Verification items for the finished model (mm, model axes). A direction names the side the tool comes from. Coordinates: 2 decimals unless noted, no trailing zeros. Order: outer loops, then holes, each group sorted by start corner. A loop starts at its lowest first (then second) coordinate and runs counter-clockwise, first axis right, second up. Notation, with made-up numbers: (45.25, -36.5) -> (98.25, -36.5) arc R33 ccw to (98.25, -8.5) -> close; hole circle Ø4 at (57, 69). An arc over 180 degrees is marked (long way). Write item = value, one per line. Start each with the question number.
Autodesk Inventor part; units mm, degrees
ref_plane "YZ Plane" through (0, 0, 0) normal (1, 0, 0) x (0, 1, 0)
ref_plane "XZ Plane" through (0, 0, 0) normal (0, 1, 0) x (-1, 0, 0)
ref_plane "XY Plane" through (0, 0, 0) normal (0, 0, 1) x (1, 0, 0)
sketch "Sketch1" plane through (0, 0, 0) normal (0, 1, 0) x (-1, 0, 0)
  line L0 (40, 50) -> (-40, 50)
  line L1 (-40, 50) -> (-40, -50)
  line L2 (-40, -50) -> (40, -50)
  line L3 (40, -50) -> (40, 50)
  line L4 (40, 50) -> (-40, -50) construction
  line L5 (-40, 50) -> (40, -50) construction
  point P0 (0, 0)
  dimension "box_width" = 80
  dimension "box_height" = 100
extrude "Base" add sketch "Sketch1" against normal blind 1.5
sketch "Sketch2" plane through (0, 0, 0) normal (0, 1, 0) x (-1, 0, 0)
  line L0 (40, -50) -> (-40, -50)
  line L1 (40, 50) -> (-40, 50)
  line L2 (-40, 50) -> (-40, -50)
  line L3 (-40, -50) -> (40, -50)
  line L4 (40, -50) -> (40, 50)
  line L5 (40, 50) -> (-40, -50) construction
  line L6 (-40, 50) -> (40, -50) construction
  line L7 (38.8, 48.5) -> (-38.8, 48.5)
  line L8 (-38.8, 48.5) -> (-38.8, -48.5)
  line L9 (-38.8, -48.5) -> (38.8, -48.5)
  line L10 (38.8, -48.5) -> (38.8, 48.5)
  line L11 (38.8, 48.5) -> (-38.8, -48.5) construction
  line L12 (-38.8, 48.5) -> (38.8, -48.5) construction
  point P0 (0, 0)
  dimension "wall_thickness" = 1.5
extrude "Wall" add sketch "Sketch2" along normal blind 50
sketch "Sketch3" plane through (0, 0, 0) normal (0, 1, 0) x (-1, 0, 0)
  line L0 (-9.25, 49) -> (9.25, 49)
  line L1 (9.25, 49) -> (9.25, 12.2)
  line L2 (9.25, 12.2) -> (-9.25, 12.2)
  line L3 (-9.25, 12.2) -> (-9.25, 49)
  line L4 (-9.25, 49) -> (9.25, 12.2) construction
  line L5 (9.25, 49) -> (-9.25, 12.2) construction
  line L6 (0, 30.6) -> (0, 0) construction
  line L7 (10.25, 50) -> (-10.25, 50)
  line L8 (-10.25, 50) -> (-10.25, 11.2)
  line L9 (-10.25, 11.2) -> (10.25, 11.2)
  line L10 (10.25, 11.2) -> (10.25, 50)
  line L11 (10.25, 50) -> (-10.25, 11.2) construction
  line L12 (-10.25, 50) -> (10.25, 11.2) construction
  line L13 (40, 50) -> (-40, 50)
  point P0 (0, 50)
  dimension "d7" = 36.8
  dimension "d8" = 18.5
  dimension "d9" = 1
  dimension "d10" = 1
extrude "Teensy Wall" add sketch "Sketch3" along normal blind 10
sketch "Sketch4" plane through (40, -1.5, -50) normal (0, 0, -1) x (-1, 0, 0)
  line L0 (78.8, 51.5) -> (1.2, 51.5) construction
  line L1 (1.2, 51.5) -> (78.8, 51.5) construction
  line L2 (40, 51.5) -> (40, 15) construction
  line L3 (40, 15) -> (20, 15) construction
  circle A0 centre (20, 15) radius 6
  line L4 (40, 15) -> (40, 0) construction
  line L5 (80, 0) -> (0, 0) construction
  circle A1 centre (40, 15) radius 6
  circle A2 centre (60, 15) radius 6
  dimension "d21" = 12
  dimension "d23" = 20
  dimension "d59" = 20
extrude "BNC Holes" cut sketch "Sketch4" against normal up to surface (1.5 mm away)
sketch "Sketch7" plane through (-38.8, 0, -48.5) normal (0, 0, 1) x (1, 0, 0)
  line L0 (78.8, 50) -> (-1.2, 50)
  line L1 (-1.2, -1.5) -> (-1.2, 50)
  line L2 (-1.2, 50) -> (-1.2, 25) construction
  line L3 (-1.2, 25) -> (13.8, 25)
  line L4 (13.8, 25) -> (-1.2, 15)
  line L5 (-1.2, 15) -> (-1.2, 25)
  line L6 (38.8, 50) -> (38.8, 0) construction
  line L7 (78.8, -1.5) -> (78.8, 50)
  line L8 (78.8, 50) -> (78.8, 25) construction
  line L9 (78.8, 25) -> (63.8, 25)
  line L10 (63.8, 25) -> (78.8, 15)
  line L11 (78.8, 15) -> (78.8, 25)
  point P0 (-1.2, 30)
  dimension "d32" = 25
  dimension "d33" = 10
  dimension "d34" = 15
extrude "Battery Support" add sketch "Sketch7" along normal up to next
sketch "Sketch8" plane through (-40, -1.5, 50) normal (0, 0, 1) x (1, 0, 0)
  line L0 (78.8, 51.5) -> (1.2, 51.5) construction
  line L1 (40, 51.5) -> (40, 1.5) construction
  line L2 (35.5, 3.5) -> (44.5, 3.5)
  line L3 (44.5, 3.5) -> (44.5, 7.5)
  line L4 (44.5, 7.5) -> (35.5, 7.5)
  line L5 (35.5, 7.5) -> (35.5, 3.5)
  line L6 (35.5, 3.5) -> (44.5, 7.5) construction
  line L7 (44.5, 3.5) -> (35.5, 7.5) construction
  point P0 (40, 5.5)
  dimension "d36" = 9
  dimension "d37" = 4
  dimension "d38" = 2
extrude "USB Hole" cut sketch "Sketch8" against normal up to next
sketch "Sketch9" plane through (-38.8, 25, -48.5) normal (0, 1, 0) x (1, 0, 0)
  line L0 (0, -97) -> (0, 0)
  line L1 (13.8, 0) -> (13.8, -97)
  line L2 (0, -79.5) -> (13.8, -79.5)
  line L3 (13.8, -79.5) -> (13.8, -78)
  line L4 (13.8, -78) -> (0, -78)
  line L5 (0, -78) -> (0, -79.5)
  line L6 (0, 0) -> (77.6, 0)
  line L7 (63.8, 0) -> (63.8, -97)
  line L8 (63.8, -79.5) -> (77.6, -79.5)
  line L9 (77.6, -79.5) -> (77.6, -78)
  line L10 (77.6, -78) -> (63.8, -78)
  line L11 (63.8, -78) -> (63.8, -79.5)
  line L12 (0, -97) -> (28.55, -97)
  line L13 (0, -79.5) -> (1.5, -79.5)
  line L14 (1.5, -79.5) -> (1.5, -97)
  line L15 (1.5, -97) -> (0, -97)
  line L16 (0, -97) -> (0, -79.5)
  line L17 (49.05, -97) -> (77.6, -97)
  line L18 (77.6, -79.5) -> (76.1, -79.5)
  line L19 (76.1, -79.5) -> (76.1, -97)
  line L20 (76.1, -97) -> (77.6, -97)
  line L21 (77.6, -97) -> (77.6, -79.5)
  line L22 (77.6, 0) -> (77.6, -97)
  line L23 (76.1, -79.5) -> (70.1, -79.5)
  line L24 (70.1, -79.5) -> (70.1, -85.5)
  line L25 (70.1, -85.5) -> (76.1, -85.5)
  line L26 (76.1, -85.5) -> (76.1, -79.5)
  line L27 (0, -78) -> (1.5, -78)
  line L28 (1.5, -78) -> (1.5, 0)
  line L29 (1.5, 0) -> (0, 0)
  line L30 (0, 0) -> (0, -78)
  line L31 (77.6, -78) -> (76.1, -78)
  line L32 (76.1, -78) -> (76.1, 0)
  line L33 (76.1, 0) -> (77.6, 0)
  line L34 (77.6, 0) -> (77.6, -78)
  line L35 (76.1, -78) -> (70.1, -78)
  line L36 (70.1, -78) -> (70.1, -72)
  line L37 (70.1, -72) -> (76.1, -72)
  line L38 (76.1, -72) -> (76.1, -78)
  line L39 (77.6, 0) -> (0, 0)
  line L40 (1.5, 0) -> (6.9705, 0)
  line L41 (1.5, -6.3005) -> (1.5, 0)
  line L42 (1.5, -78) -> (6.9, -78)
  line L43 (1.5, -72.6667) -> (1.5, -78)
  line L44 (1.5, -78) -> (6.9, -78)
  line L45 (1.5, -72) -> (1.5, -78)
  line L46 (1.5, -78) -> (7.5, -78)
  line L47 (7.5, -78) -> (7.5, -72)
  line L48 (7.5, -72) -> (1.5, -72)
  line L49 (1.5, -72) -> (1.5, -78)
  point P0 (38.8, -48.5)
  dimension "d41" = 78
  dimension "d42" = 1.5
  dimension "d45" = 1.5
  dimension "d47" = 1.5
  dimension "d48" = 6
  dimension "d56" = 17.5
extrude "Plate Support" add sketch "Sketch9" along normal blind 23.5 contours L0 L2 L14 L12 | L0 L4 L1 L2 | L0 L6 L28 L4 | L28 L48 L47 L4 | L6 L22 L10 L32 | L10 L9 L8 L7 | L32 L10 L36 L37 | L8 L19 L25 L24 | L21 L17 L19 L8
sketch "Sketch10" plane through (-38.8, 48.5, -48.5) normal (0, 1, 0) x (1, 0, 0)
  circle A0 centre (73.1, -82.5) radius 1.45
  line L0 (63.8, -78) -> (70.1, -78) construction
  line L1 (70.1, -85.5) -> (70.1, -79.5) construction
  line L2 (70.1, -79.5) -> (73.1, -82.5) construction
  line L3 (70.1, -85.5) -> (76.1, -85.5) construction
  line L4 (73.1, -82.5) -> (76.1, -85.5) construction
  line L5 (73.1, -82.5) -> (70.1, -85.5) construction
  circle A1 centre (73.1, -75) radius 1.45
  line L6 (73.1, -75) -> (70.1, -72) construction
  line L7 (70.1, -72) -> (76.1, -72) construction
  line L8 (76.1, -72) -> (73.1, -75) construction
  line L9 (70.1, -78) -> (73.1, -75) construction
  line L10 (1.5, -72) -> (1.5, 0)
  line L11 (1.5, -78) -> (7.5, -78)
  line L12 (7.5, -78) -> (7.5, -72)
  line L13 (7.5, -72) -> (1.5, -72)
  line L14 (1.5, -72) -> (1.5, -78)
  line L15 (70.1, -72) -> (70.1, -78)
  circle A2 centre (4.5, -75) radius 1.45
  line L16 (7.5, -78) -> (7.5, -72) construction
  line L17 (4.5, -75) -> (7.5, -78) construction
  line L18 (4.5, -75) -> (7.5, -72) construction
  line L19 (4.5, -75) -> (1.5, -72) construction
  point P0 (38.8, -48.5)
  dimension "d49" = 2.9
  dimension "d52" = 2.9
  dimension "d53" = 2.9
extrude "Holes" cut sketch "Sketch10" against normal blind 10 contours A0 | A1 | A2
sketch "Sketch11" plane through (-38.8, 48.5, -48.5) normal (0, 1, 0) x (1, 0, 0)
  line L0 (13.8, -79.5) -> (13.8, -78)
  line L1 (13.8, -78) -> (13.8, -79.5)
  line L2 (13.8, -79.5) -> (0.1333, -79.5)
  line L3 (0.1333, -79.5) -> (0.1333, -78)
  line L4 (0.1333, -78) -> (13.8, -78)
  line L5 (70.1, -78) -> (63.8, -78)
  line L6 (63.8, -78) -> (63.8, -79.5)
  line L7 (63.8, -79.5) -> (77.4667, -79.5)
  line L8 (77.4667, -79.5) -> (77.4667, -78)
  line L9 (77.4667, -78) -> (63.8, -78)
  point P0 (38.8, -48.5)
extrude "Extrusion10" add sketch "Sketch11" along normal blind 1.5
properties part number "teensy_box"
Item 1: Thickness scan on line 1 (X direction, y = 13, z = -49); line 2 (Z direction, x = -30, y = 37.5); line 3 (Z direction, x = -36.5, y = 28). Record the ranges inside material, lowest first.
Item 2: Section check B-B (y = 34). Record the boundary of the cut face in (x, z).
Item 3: Tool access check on faces 1 (the cylindrical face through (24.76, 9.85, -49.26)), 2 (the flat face through (-1, 25, 50)), 3 (the flat face through (9.25, 5, 30)), 4 (the flat face through (1, 25, -48.5)), 5 (the flat face through (1, 25, -50)). Record the directions out of +Z, -Z, +X, -X, +Y, -Y that give a thin tool (end or side, any length) a straight path to the whole face; none if there is none.
Item 4: Gauge pin test, flat ends, axial feed: P1, Ø1.4, axis at x = -34.5, z = 27, coming from the +Y side; P2, Ø12, axis at x = -14, z = -13, coming from the +Y side; P3, Ø15, axis at x = -2, z = 38, coming from the +Y side; P4, Ø11, axis at x = 4, y = 4.5, coming from the +Z side. Record the tip position at first contact, or that the pin passes through.
Item 5: Section check C-C (z = 5.5). Record the boundary of the cut face in (x, y), then the cut area to 3 significant figures.
Item 6: Mould release check, pull along Y, two halves, no side actions. Record for faces 6 (the flat face through (-1, 25, 48.5)), 7 (the flat face through (34, 38.5, 34)), 8 (the flat face through (37.3, 37, -12)): pulls with the +Y half, pulls with the -Y half, needs draft (parallel to the pull), parting line crosses it, or undercut.
Item 7: Section check D-D (x = -20). Record the boundary of the cut face in (y, z).
Item 8: Section check A-A (y = 13.5). Record the boundary of the cut face in (x, z), then the cut area to 3 significant figures.
Filled sheet:
q1.line_1 = -40 to -25.98, -14.02 to -5.98, 5.98 to 14.02, 25.98 to 40
q1.line_2 = -50 to -48.5, 29.5 to 31, 48.5 to 50
q1.line_3 = -50 to -48.5, 23.5 to 31, 48.5 to 50
q2.outline = (-40, -50) -> (40, -50) -> (40, 50) -> (-40, 50) -> close; hole (-37.3, -48.5) -> (37.3, -48.5) -> (37.3, 23.5) -> (31.3, 23.5) -> (31.3, 29.5) -> (25, 29.5) -> (25, 31) -> (31.3, 31) -> (31.3, 37) -> (37.3, 37) -> (37.3, 48.5) -> (-37.3, 48.5) -> (-37.3, 31) -> (-25, 31) -> (-25, 29.5) -> (-31.3, 29.5) -> (-31.3, 23.5) -> (-37.3, 23.5) -> close
q3.face_1 = -Z
q3.face_2 = +Z, +X, -X, +Y, -Y
q3.face_3 = +Y
q3.face_4 = none
q3.face_5 = -Z, +X, -X, +Y, -Y
q4.P1 = 38.5
q4.P2 = 0
q4.P3 = 10
q4.P4 = 50
q5.outline = (-40, -1.5) -> (40, -1.5) -> (40, 50) -> (38.8, 50) -> (38.8, 48.5) -> (37.3, 48.5) -> (37.3, 25) -> (25, 25) -> (38.8, 15.8) -> (38.8, 0) -> (-38.8, 0) -> (-38.8, 15.8) -> (-25, 25) -> (-37.3, 25) -> (-37.3, 48.5) -> (-38.8, 48.5) -> (-38.8, 50) -> (-40, 50) -> close
q5.area = 437 mm^2
q6.face_6 = undercut
q6.face_7 = pulls with the +Y half
q6.face_8 = needs draft
q7.outline = (-1.5, -50) -> (7.5, -50) -> (7.5, -48.5) -> (0, -48.5) -> (0, 48.5) -> (50, 48.5) -> (50, 50) -> (-1.5, 50) -> close; (19.5, -50) -> (50, -50) -> (50, -48.5) -> (19.5, -48.5) -> close
q8.outline = (-40, -50) -> (-26, -50) -> (-26, -48.5) -> (-38.8, -48.5) -> (-38.8, 48.5) -> (38.8, 48.5) -> (38.8, -48.5) -> (26, -48.5) -> (26, -50) -> (40, -50) -> (40, 50) -> (-40, 50) -> close; (-14, -50) -> (-6, -50) -> (-6, -48.5) -> (-14, -48.5) -> close; (6, -50) -> (14, -50) -> (14, -48.5) -> (6, -48.5) -> close
q8.area = 419 mm^2
